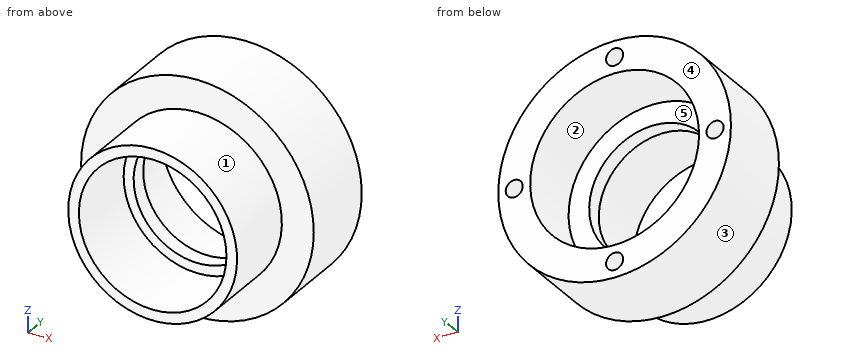
```python
from build123d import *

# Parameters (mm, degrees)
SKETCH1_R                      = 7.9375
SKETCH1_R_2                    = 6.9375
BOSS_EXTRUDE1_DEPTH            = 7
SKETCH2_R                      = 7.9375
SKETCH2_R_2                    = 6
BOSS_EXTRUDE2_DEPTH            = 1.5
SKETCH3_R                      = 10.9375
SKETCH3_R_2                    = 7.9375
BOSS_EXTRUDE3_DEPTH            = 6
M2X0_4_TAPPED_HOLE1_AT_2_COUNT = 2
M2X0_4_TAPPED_HOLE1_AT_2_PITCH = 13.346640495
M2X0_4_TAPPED_HOLE1_AT_3_COUNT = 2
M2X0_4_TAPPED_HOLE1_AT_3_PITCH = 18.875
M2X0_4_TAPPED_HOLE1_AT_4_COUNT = 2
M2X0_4_TAPPED_HOLE1_AT_4_PITCH = 13.346640495
BOSS_EXTRUDE4_START            = 1.5
SKETCH7_R                      = 10.9375
SKETCH7_R_2                    = 6.9375
BOSS_EXTRUDE4_DEPTH            = 1.5


with BuildPart() as part:
    # Sketch1 → Boss-Extrude1 (new body)
    with BuildSketch(Plane(origin=(0, 0, 0), x_dir=(1, 0, 0), z_dir=(0, 1, 0))):
        with Locations(Location((0, 0, 0), (0, 0, 270))):
            Circle(SKETCH1_R)
        with Locations(Location((0, 0, 0), (0, 0, 270))):
            Circle(SKETCH1_R_2, mode=Mode.SUBTRACT)
    extrude(amount=BOSS_EXTRUDE1_DEPTH)

    # Sketch2 → Boss-Extrude2 (add)
    with BuildSketch(Plane(origin=(0, 7, 0), x_dir=(1, 0, 0), z_dir=(0, 1, 0))):
        with Locations(Location((0, 0, 0), (0, 0, 270))):
            Circle(SKETCH2_R)
        with Locations(Location((0, 0, 0), (0, 0, 270))):
            Circle(SKETCH2_R_2, mode=Mode.SUBTRACT)
    extrude(amount=BOSS_EXTRUDE2_DEPTH)



with BuildPart() as body_2:
    # Sketch3 → Boss-Extrude3 (new body)
    with BuildSketch(Plane(origin=(0, 8.5, 0), x_dir=(1, 0, 0), z_dir=(0, 1, 0))):
        with Locations(Location((0, 0, 0), (0, 0, 270))):
            Circle(SKETCH3_R)
        with Locations(Location((0, 0, 0), (0, 0, 270))):
            Circle(SKETCH3_R_2, mode=Mode.SUBTRACT)
    extrude(amount=BOSS_EXTRUDE3_DEPTH)

    # Sketch5 → M2x0.4 Tapped Hole1 (revolve, cut)
    with BuildSketch(Plane(origin=(0, 14.5, -9.4375), x_dir=(0, 0, 1), z_dir=(1, 0, 0))):
        Polygon((0, 0), (0, 6.180688495), (0.8, 5.7), (0.8, 0), align=None)
    m2x0_4_tapped_hole1 = revolve(axis=Axis((0, 20.85, -9.4375), (0, -1, 0)), mode=Mode.SUBTRACT)

    # M2x0.4 Tapped Hole1 at 2: M2x0.4 Tapped Hole1 ×2
    with Locations(*[Vector(0.7071067811865476, 0, 0.7071067811865476) * (i * M2X0_4_TAPPED_HOLE1_AT_2_PITCH) for i in range(1, M2X0_4_TAPPED_HOLE1_AT_2_COUNT)]):
        add(m2x0_4_tapped_hole1, mode=Mode.SUBTRACT)

    # M2x0.4 Tapped Hole1 at 3: M2x0.4 Tapped Hole1 ×2
    with Locations(*[(0, 0, i * M2X0_4_TAPPED_HOLE1_AT_3_PITCH) for i in range(1, M2X0_4_TAPPED_HOLE1_AT_3_COUNT)]):
        add(m2x0_4_tapped_hole1, mode=Mode.SUBTRACT)

    # M2x0.4 Tapped Hole1 at 4: M2x0.4 Tapped Hole1 ×2
    with Locations(*[Vector(-0.7071067811865476, 0, 0.7071067811865476) * (i * M2X0_4_TAPPED_HOLE1_AT_4_PITCH) for i in range(1, M2X0_4_TAPPED_HOLE1_AT_4_COUNT)]):
        add(m2x0_4_tapped_hole1, mode=Mode.SUBTRACT)


with BuildPart() as part_1:
    add(part.part)

    add(body_2.part)  # Boss-Extrude4 merges body 2
    # Sketch7 → Boss-Extrude4 (add)
    with BuildSketch(Plane.XZ.offset(-8.5).offset(BOSS_EXTRUDE4_START)):
        with Locations(Location((0, 0, 0), (0, 0, 90))):
            Circle(SKETCH7_R)
        with Locations(Location((0, 0, 0), (0, 0, 90))):
            Circle(SKETCH7_R_2, mode=Mode.SUBTRACT)
    extrude(amount=-BOSS_EXTRUDE4_DEPTH)


solid = part_1.part
```
CAD build for the part. Positions are in the model's coordinates, mm. Face numbers are marked on the shaded views. A direction names the side the tool comes from. Coordinates: 2 decimals unless noted, no trailing zeros. Write each loop counter-clockwise with the first axis right and the second up, starting at its lowest first coordinate (ties: lowest second). Pieces come first, ordered by that corner, then holes. Notation, with made-up numbers: (40, 21.5) -> (57, 21.5) arc R30 cw to (57, 46.5) -> close; hole circle Ø11 at (15.25, -15.75). An arc over 180 degrees is marked (long way). Return JSON: item names as keys, results as strings. Group by question number.
Q1. Pull direction Z, two halves, no side cores. Call the marked faces 3, 4 and 5: released by +Z, released by -Z, zero draft, split by the parting line, or undercut.
Q2. Which spindle directions (+Z, -Z, +X, -X, +Y, -Y) get a long thin tool onto all of the face, cutting with end or side? Do the marked faces 1 and 2. Say none if no direction does.
Q3. Drill centre lines: line 1 (X direction, y = 11.25, z = 0); line 2 (X direction, y = 8.05, z = 0); line 3 (X direction, y = 3.5, z = 0). Where is each one in solid material? Low to high.
Q4. Flat gauge pins, fed straight in: pin 1 (1.4 mm diameter, centred on x = -9.44, z = 0, fed in from +Y); pin 2 (0.7 mm diameter, centred on x = 9.5, z = 0, fed in from +Y); pin 3 (1 mm diameter, centred on x = 0, z = -9.44, fed in from -Y). Where does each tip first touch, or does it go through?
Q5. Cut at D-D, the plane y = 12.75. Give the cut face in (x, z) (1 decimal), then the cut area to 3 significant figures.
Q6. Cut at C-C, the plane y = 6.5. Give the cut face in (x, z) (1 decimal), then the cut area to 3 significant figures.
Returned:
{
 "1": {"face 3": "split by the parting line", "face 4": "zero draft", "face 5": "undercut"},
 "2": {"face 1": "-Y", "face 2": "+Y"},
 "3": {"line 1": "x = -10.94 to -10.24, -8.64 to -7.94, 7.94 to 8.64, 10.24 to 10.94", "line 2": "x = -10.94 to -6, 6 to 10.94", "line 3": "x = -7.94 to -6.94, 6.94 to 7.94"},
 "4": {"pin 1": "stops at y = 8.74", "pin 2": "stops at y = 8.57", "pin 3": "stops at y = 7"},
 "5": {"outline": "circle Ø21.9 at (0, 0); hole circle Ø1.6 at (-9.4, 0); hole circle Ø15.9 at (0, 0); hole circle Ø1.6 at (0, -9.4); hole circle Ø1.6 at (0, 9.4); hole circle Ø1.6 at (9.4, 0)", "area": "170 mm2"},
 "6": {"outline": "circle Ø15.9 at (0, 0); hole circle Ø13.9 at (0, 0)", "area": "46.7 mm2"}
}
